```python
from build123d import *

# Parameters (mm, degrees)
F0_R     = 10
F1_DEPTH = 25
F2_DEPTH = 50
F3_SIZE  = 2
F5_R     = 12.5
F6_DEPTH = 25.001


with BuildPart() as f1:
    # F0 (on Front) → F1 (new body)
    with BuildSketch(Plane.XZ):
        with BuildLine():
            ThreePointArc((2.083333, -24.913043), (18.399502, -16.92508), (25, 0))
            ThreePointArc((25, 0), (18.399502, 16.92508), (2.083333, 24.913043))
            ThreePointArc((2.083333, 24.913043), (-25, 0), (2.083333, -24.913043))
        make_face()
        Circle(F0_R, mode=Mode.SUBTRACT)
        with BuildLine():
            ThreePointArc((2.083333, 24.913043), (18.399502, 16.92508), (25, 0))
            ThreePointArc((25, 0), (18.399502, -16.92508), (2.083333, -24.913043))
            Line((2.083333, -24.913043), (91.458333, -17.43913))
            ThreePointArc((91.458333, -17.43913), (72.5, 0), (91.458333, 17.43913))
            Line((91.458333, 17.43913), (2.083333, 24.913043))
        make_face()
        with BuildLine():
            ThreePointArc((107.5, 0), (102.879651, 11.847556), (91.458333, 17.43913))
            ThreePointArc((91.458333, 17.43913), (72.5, 0), (91.458333, -17.43913))
            ThreePointArc((91.458333, -17.43913), (102.879651, -11.847556), (107.5, 0))
        make_face()
        with Locations((90, 0)):
            Circle(F0_R, mode=Mode.SUBTRACT)
    extrude(amount=F1_DEPTH)

    # F0 (on Front) → F2 (join)
    with BuildSketch(Plane.XZ):
        with BuildLine():
            ThreePointArc((2.083333, -24.913043), (18.399502, -16.92508), (25, 0))
            ThreePointArc((25, 0), (18.399502, 16.92508), (2.083333, 24.913043))
            ThreePointArc((2.083333, 24.913043), (-25, 0), (2.083333, -24.913043))
        make_face()
        Circle(F0_R, mode=Mode.SUBTRACT)
    extrude(amount=F2_DEPTH)

    # F3
    f3_edges = [f1.edges().sort_by_distance(p)[0] for p in [
        (-2.083333, -50, 24.913043),
        (-10, -50, 0),
        (80, -25, 0),
    ]]
    chamfer(f3_edges, length=F3_SIZE)

    # F5 (on face) → F6 (cut, through all)
    with BuildSketch(Plane.XZ.offset(25)):
        with Locations((48.291023, 0)):
            Circle(F5_R)
    extrude(amount=-F6_DEPTH, mode=Mode.SUBTRACT)


solid = f1.part
```
Geometry check sheet. Reference: the model listing, model coordinates, mm. Give positions to 0.01 mm unless a question says otherwise; leave off trailing zeros. Order: outer loops, then holes, each group sorted by start corner. A loop starts at its lowest first (then second) coordinate and runs counter-clockwise, first axis right, second up. Notation, with made-up numbers: (4.25, 89) - (20.25, 89) arc R29 ccw to (20.25, 116) - close; hole circle Ø10 at (-23, 13.25). An arc over 180 degrees is marked (long way). Answer in a Markdown table with one row per item. Add a question column.
Q1. Cross-section at C-C, the plane y = -38.5. Enter the section's corners in (x, z).
Q2. Cross-section at B-B, the plane x = 0. Enter the section's corners in (y, z).
Q3. Gauge pin test, flat ends, axial feed: pin 1 (6 mm diameter, centred on y = -40, z = -19.5, fed in from -X); pin 2 (2 mm diameter, centred on y = -14, z = -5.5, fed in from +X); pin 3 (10 mm diameter, centred on x = 32.5, z = -15.5, fed in from -Y). Record the tip position at first contact, or that the pin passes through.
Q4. Mould release check, pull along X, two halves, no side actions. Record for faces 1 (the conical face through (81.965, -23.125, -6.161)), 2 (the flat face through (46.15, -12.32, -21.23)), 3 (the flat face through (66, -25, 0)): pulls with the +X half, pulls with the -X half, needs draft (parallel to the pull), parting line crosses it, or undercut.
Q5. Material ranges on probe 1 along X at (y, z) = (-20, -4); probe 2 along Z at (x, y) = (0, -25.5); probe 3 along Y at (x, z) = (20.5, -15.5), recorded low to high. Write a range as from..to.
Q6. Cross-section at D-D, the plane x = 54. Enter the section's corners in (y, z), then the cut area to 3 significant figures.
Q7. Cross-section at A-A, the plane y = -9. Enter the section's corners in (x, z).
Check values:
| question | item | result |
|---|---|---|
| 1 | outline | (2.08, -24.91) arc R25 ccw to (25, 0) arc R25 ccw to (2.08, 24.91) arc R25 ccw (long way) to start; hole circle Ø20 at (0, 0) |
| 2 | outline | (-50, -23) - (-48, -25) - (0, -25) - (0, -10) - (-48, -10) - (-50, -12) - close; (-50, 12) - (-48, 10) - (0, 10) - (0, 25) - (-48, 25) - (-50, 23) - close |
| 3 | pin 1 | stops at x = -18.78 |
| 3 | pin 2 | stops at x = 106.91 |
| 3 | pin 3 | stops at y = -25 |
| 4 | face 1 | undercut |
| 4 | face 2 | pulls with the +X half |
| 4 | face 3 | needs draft |
| 5 | probe 1 | x = -24.68..-9.17, 9.17..36.45, 60.13..80.83, 99.17..107.04 |
| 5 | probe 2 | z = -25..-10, 10..25 |
| 5 | probe 3 | y = -25..0 |
| 6 | outline | (-25, -20.57) - (0, -20.57) - (0, -11.12) - (-25, -11.12) - close; (-25, 11.12) - (0, 11.12) - (0, 20.57) - (-25, 20.57) - close |
| 6 | area | 473 mm^2 |
| 7 | outline | (2.08, -24.91) - (91.46, -17.44) arc R17.5 ccw to (91.46, 17.44) - (2.08, 24.91) arc R25 ccw (long way) to start; hole circle Ø20 at (0, 0); hole circle Ø25 at (48.29, 0); hole circle Ø20 at (90, 0) |
